Study the drawing (mm; zero at the part's minimum x, y, z) and answer. A direction names the side the tool comes from. Round coordinates to 2 decimals unless told otherwise and drop trailing zeros. Write each loop counter-clockwise with the first axis right and the second up, starting at its lowest first coordinate (ties: lowest second). Pieces come first, ordered by that corner, then holes. Notation, with made-up numbers: (78.5, 34) -> (97.5, 34) arc R18 cw to (97.5, 53) -> close; hole circle Ø7 at (80.25, 29). An arc over 180 degrees is marked (long way). Return JSON: item names as keys, results as strings.
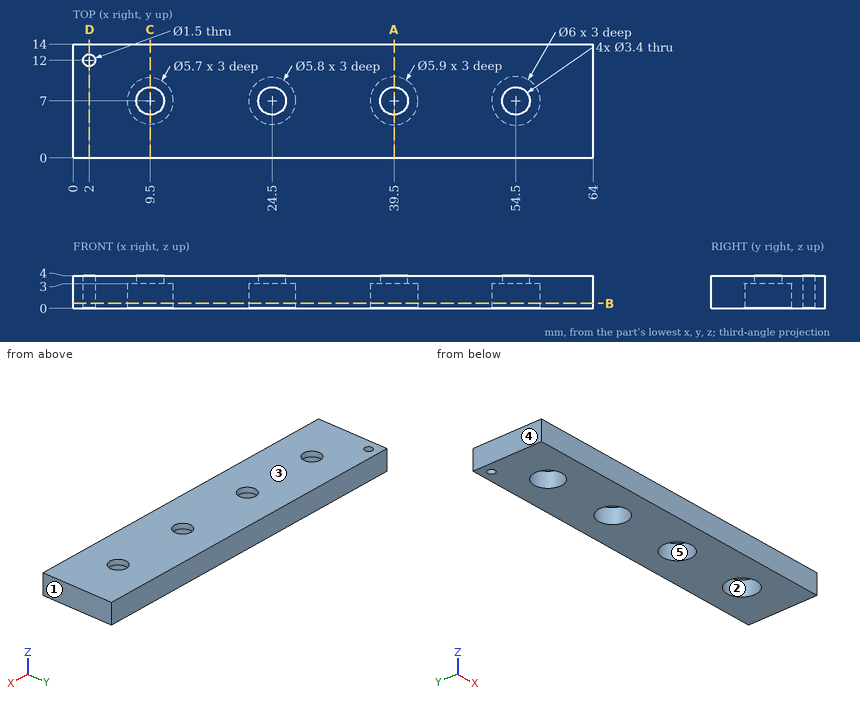
Item 1: For a pull along X with two mould halves and no side action, classify the marked faces 1, 2 and 3 as released by +X, released by -X, zero draft, split by the parting line, or undercut.
Worked answers:
{"face 1": "released by +X", "face 2": "undercut", "face 3": "zero draft"}
Item 2: Section A-A (x = 39.5) is taken. Give the vertices of the cut face in (y, z), then the cut area to 3 significant figures.
Worked answers:
{"outline": "(0, 0) -> (4.05, 0) -> (4.05, 3) -> (5.3, 3) -> (5.3, 4) -> (0, 4) -> close; (8.7, 3) -> (9.95, 3) -> (9.95, 0) -> (14, 0) -> (14, 4) -> (8.7, 4) -> close", "area": "34.9 mm2"}
Item 3: Flat-ended cylindrical pins translate along their axes: pin 1 (8 mm diameter, centred on x = 54.5, y = 7, fed in from +Z); pin 2 (4.5 mm diameter, centred on x = 39.5, y = 7, fed in from -Z); pin 3 (3 mm diameter, centred on x = 54.5, y = 7, fed in from +Z). Find the tip coordinate at first contact, or state that the pin passes through.
Worked answers:
{"pin 1": "stops at z = 4", "pin 2": "stops at z = 3", "pin 3": "passes through"}
Item 4: Straight lines are drawn through the part: L1, parallel to X at y = 6.75, z = 1.85; L2, parallel to X at y = 7, z = 3.6; L3, parallel to Y at x = 54.5, z = 2.45. For each, find the intervals that lie inside material, in ascending order. Write a range as [from, to].
Worked answers:
{"L1": "x = [0, 6.66], [12.34, 21.61], [27.39, 36.56], [42.44, 51.51], [57.49, 64]", "L2": "x = [0, 7.8], [11.2, 22.8], [26.2, 37.8], [41.2, 52.8], [56.2, 64]", "L3": "y = [0, 4], [10, 14]"}
Item 5: Section B-B (z = 0.6) is taken. Give the vertices of the cut face in (x, y), then the cut area to 3 significant figures.
Worked answers:
{"outline": "(0, 0) -> (64, 0) -> (64, 14) -> (0, 14) -> close; hole circle Ø1.5 at (2, 12); hole circle Ø5.7 at (9.5, 7); hole circle Ø5.8 at (24.5, 7); hole circle Ø5.9 at (39.5, 7); hole circle Ø6 at (54.5, 7)", "area": "787 mm2"}
Item 6: Section D-D (x = 2) is taken. Give the vertices of the cut face in (y, z), then the cut area to 3 significant figures.
Worked answers:
{"outline": "(0, 0) -> (11.25, 0) -> (11.25, 4) -> (0, 4) -> close; (12.75, 0) -> (14, 0) -> (14, 4) -> (12.75, 4) -> close", "area": "50.0 mm2"}
Item 7: Section C-C (x = 9.5) is taken. Give the vertices of the cut face in (y, z).
Worked answers:
{"outline": "(0, 0) -> (4.15, 0) -> (4.15, 3) -> (5.3, 3) -> (5.3, 4) -> (0, 4) -> close; (8.7, 3) -> (9.85, 3) -> (9.85, 0) -> (14, 0) -> (14, 4) -> (8.7, 4) -> close"}
Item 8: A tool of negligible diameter and unlimited length cuts with its end or side. For the marked faces 4 and 5, from which of +Z, -Z, +X, -X, +Y, -Y can it reach the whole face along a straight path? Write none if from no direction.
Worked answers:
{"face 4": "+Z, -Z, -X, +Y, -Y", "face 5": "-Z"}
